Study the drawing (mm; zero at the part's minimum x, y, z) and answer. Give positions to 0.01 mm unless a question says otherwise; leave off trailing zeros. Loops run counter-clockwise (first coordinate to the right, second up) from the corner with the lowest first, then second, coordinate; pieces in that order, holes last. Notation, with made-up numbers: (67, 55.5) - (114, 55.5) arc R16 ccw to (114, 81.5) - close; hole circle Ø8 at (-32, 32.5). An arc over 180 degrees is marked (long way). Write item = value, one per line. Start each with the question number.
1) The part is cut by section C-C on y = 6.75. Write down the section's boundary in (x, z).
2) The part is cut by section D-D on x = 18. Write down the section's boundary in (y, z) (1 decimal), plus the area to 3 significant figures.
3) The part is cut by section B-B on z = 3.85. Write down the section's boundary in (x, y) (1 decimal), plus the area to 3 significant figures.
4) Consider probe 1 along Y at (x, z) = (26, 3.3); probe 2 along Y at (x, z) = (18.5, 4.6). Determine where each line is inside the solid, lowest interval first.
5) The mould has two halves that part along X. Classify the marked faces 1, 2 and 3: +X half, -X half, draft (parallel to the pull), parting line (faces both ways), or undercut.
6) The part is cut by section A-A on y = 2.5. Write down the section's boundary in (x, z).
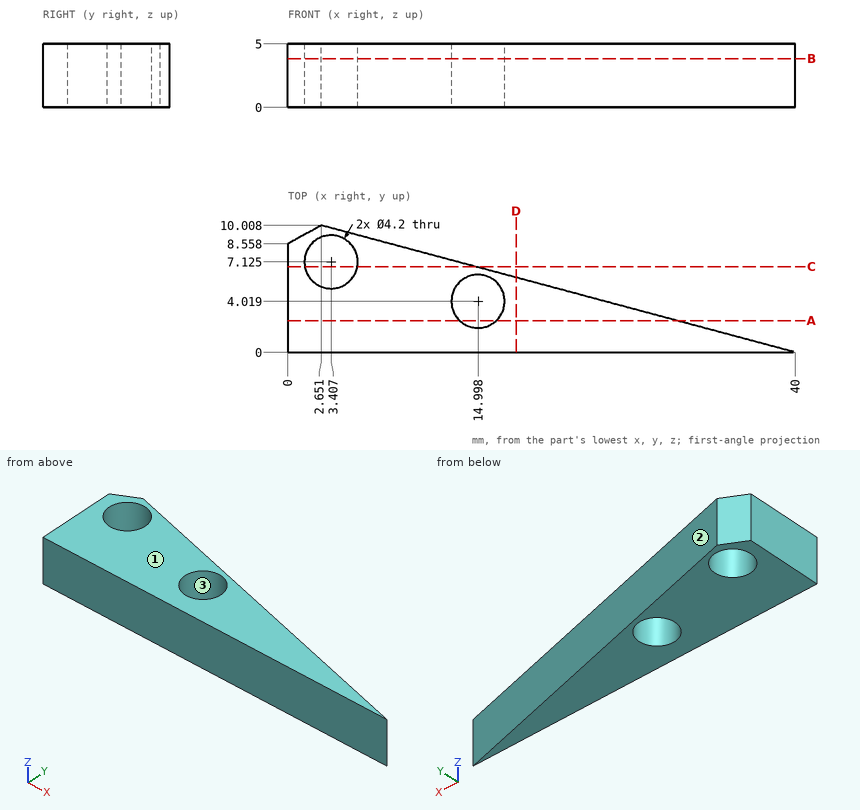
Answer below:
q1.outline = (0, 0) - (1.34, 0) - (1.34, 5) - (0, 5) - close; (5.47, 0) - (14.81, 0) - (14.81, 5) - (5.47, 5) - close
q2.outline = (0, 0) - (5.9, 0) - (5.9, 5) - (0, 5) - close
q2.area = 29.5 mm2
q3.outline = (0, 0) - (40, 0) - (2.7, 10) - (0, 8.6) - close; hole circle Ø4.2 at (3.4, 7.1); hole circle Ø4.2 at (15, 4)
q3.area = 184 mm2
q4.probe_1 = 0 to 3.75
q4.probe_2 = 0 to 5.76
q5.face_1 = draft
q5.face_2 = +X half
q5.face_3 = undercut
q6.outline = (0, 0) - (13.55, 0) - (13.55, 5) - (0, 5) - close; (16.45, 0) - (30.67, 0) - (30.67, 5) - (16.45, 5) - close
